Could you check a few things on this model? Use its own coordinates, in mm. A direction names the side the tool comes from. Round coordinates to 2 decimals unless told otherwise and drop trailing zeros. Write each loop counter-clockwise with the first axis right and the second up, starting at its lowest first coordinate (ties: lowest second). Pieces come first, ordered by that corner, then holes. Notation, with made-up numbers: (-22, 62) -> (31, 62) arc R9 cw to (31, 72) -> close; hole circle Ø5 at (-22, 82). An arc over 180 degrees is marked (long way). Answer in a Markdown table with one row per item.
from build123d import *

# Parameters (mm, degrees)
F0_W     = 90
F0_H     = 70
F0_W_2   = 87
F0_H_2   = 67
F1_DEPTH = 25
F0_R     = 3.1
F0_R_2   = 1.025
F2_DEPTH = 1.5
F3_DEPTH = 5


with BuildPart() as f1:
    # F0 (on Top) → F1 (new body)
    with BuildSketch(Plane.XY):
        with Locations((-0.797456, -0.095572)):
            Rectangle(F0_W, F0_H)
        with Locations((-0.797456, -0.095572)):
            Rectangle(F0_W_2, F0_H_2, mode=Mode.SUBTRACT)
    extrude(amount=F1_DEPTH)

    # F0 (on Top) → F2 (join)
    with BuildSketch(Plane.XY):
        with Locations((-0.797456, -0.095572)):
            Rectangle(F0_W, F0_H)
        with Locations((-0.797456, -0.095572)):
            Rectangle(F0_W_2, F0_H_2, mode=Mode.SUBTRACT)
        with Locations((-0.797456, -0.095572)):
            Rectangle(F0_W_2, F0_H_2)
        with Locations((-19.797456, -27.095572)):
            Circle(F0_R, mode=Mode.SUBTRACT)
        with Locations((38.202544, -27.095572)):
            Circle(F0_R, mode=Mode.SUBTRACT)
        with Locations((-19.797456, 21.904428)):
            Circle(F0_R, mode=Mode.SUBTRACT)
        with Locations((38.202544, 21.904428)):
            Circle(F0_R, mode=Mode.SUBTRACT)
        with Locations((38.202544, -27.095572)):
            Circle(F0_R)
        with Locations((38.202544, -27.095572)):
            Circle(F0_R_2, mode=Mode.SUBTRACT)
        with Locations((38.202544, -27.095572)):
            Circle(F0_R_2)
        with Locations((38.202544, 21.904428)):
            Circle(F0_R)
        with Locations((38.202544, 21.904428)):
            Circle(F0_R_2, mode=Mode.SUBTRACT)
        with Locations((38.202544, 21.904428)):
            Circle(F0_R_2)
        with Locations((-19.797456, 21.904428)):
            Circle(F0_R)
        with Locations((-19.797456, 21.904428)):
            Circle(F0_R_2, mode=Mode.SUBTRACT)
        with Locations((-19.797456, 21.904428)):
            Circle(F0_R_2)
        with Locations((-19.797456, -27.095572)):
            Circle(F0_R)
        with Locations((-19.797456, -27.095572)):
            Circle(F0_R_2, mode=Mode.SUBTRACT)
        with Locations((-19.797456, -27.095572)):
            Circle(F0_R_2)
    extrude(amount=-F2_DEPTH)

    # F0 (on Top) → F3 (join)
    with BuildSketch(Plane.XY):
        with Locations((-19.797456, 21.904428)):
            Circle(F0_R)
        with Locations((-19.797456, 21.904428)):
            Circle(F0_R_2, mode=Mode.SUBTRACT)
        with Locations((38.202544, 21.904428)):
            Circle(F0_R)
        with Locations((38.202544, 21.904428)):
            Circle(F0_R_2, mode=Mode.SUBTRACT)
        with Locations((38.202544, -27.095572)):
            Circle(F0_R)
        with Locations((38.202544, -27.095572)):
            Circle(F0_R_2, mode=Mode.SUBTRACT)
        with Locations((-19.797456, -27.095572)):
            Circle(F0_R)
        with Locations((-19.797456, -27.095572)):
            Circle(F0_R_2, mode=Mode.SUBTRACT)
    extrude(amount=F3_DEPTH)


solid = f1.part
1) For faces 1 (the face through (-20, 22, 0)), 2 (the face through (-1, 0, -1.5)), which set-ups out of +Z, -Z, +X, -X, +Y, -Y let a thin tool reach every point of the face, with its end or its side?
Findings:
| item | result |
|---|---|
| face 1 | +Z |
| face 2 | -Z, +X, -X, +Y, -Y |
2) Imagine slicing it at D-D, the plane z = 14.5. Please give me the cut outline in (x, y).
Findings:
| item | result |
|---|---|
| outline | (-45.8, -35.1) -> (44.2, -35.1) -> (44.2, 34.9) -> (-45.8, 34.9) -> close; hole (-44.3, -33.6) -> (42.7, -33.6) -> (42.7, 33.4) -> (-44.3, 33.4) -> close |
3) Imagine slicing it at C-C, the plane x = 18. Please give me the cut outline in (y, z).
Findings:
| item | result |
|---|---|
| outline | (-35.1, -1.5) -> (34.9, -1.5) -> (34.9, 25) -> (33.4, 25) -> (33.4, 0) -> (-33.6, 0) -> (-33.6, 25) -> (-35.1, 25) -> close |
4) Imagine slicing it at B-B, the plane z = 1. Count the separate pieces of the cut face and the enclosed holes in it, plus the area to 3 significant figures.
Findings:
| item | result |
|---|---|
| separate pieces | 5 |
| enclosed holes | 5 |
| area | 579 mm^2 |
5) For pin 1 (3.5 mm diameter, centred on x = 38.2, y = -27.1, fed in from +Z); pin 2 (0.6 mm diameter, centred on x = -19.5, y = 22, fed in from +Z), each with a flat end and sliding along its axis, tell me the tip position at first contact or that it passes through.
Findings:
| item | result |
|---|---|
| pin 1 | stops at z = 5 |
| pin 2 | stops at z = 0 |
6) Thinking about a two-plate mould opening in Y: for faces 3 (the face through (-21, 23, 5)), 4 (the face through (39.15, 21.51, 2.46)), 5 (the face through (-45.797, -1, 12)), 6 (the face through (-1, -35.096, 12)), which applies, +Y half, -Y half, draft (parallel to the pull), parting line (faces both ways), or undercut?
Findings:
| item | result |
|---|---|
| face 3 | undercut |
| face 4 | undercut |
| face 5 | draft |
| face 6 | -Y half |
7) Please list where these lines run through material, in increasing order: line 1 (Y direction, x = -16, z = 4); line 2 (X direction, y = -27, z = 18); line 3 (Z direction, x = 34, y = 6).
Findings:
| item | result |
|---|---|
| line 1 | y = -35.1 to -33.6, 33.4 to 34.9 |
| line 2 | x = -45.8 to -44.3, 42.7 to 44.2 |
| line 3 | z = -1.5 to 0 |
8) Imagine slicing it at A-A, the plane y = 16.5. Please give me the cut outline in (x, z).
Findings:
| item | result |
|---|---|
| outline | (-45.8, -1.5) -> (44.2, -1.5) -> (44.2, 25) -> (42.7, 25) -> (42.7, 0) -> (-44.3, 0) -> (-44.3, 25) -> (-45.8, 25) -> close |
